```python
from build123d import *

# Parameters (mm, degrees)
HOLE_WIZARD_1_D           = 17.5
HOLE_WIZARD_1_DEPTH       = 23.999
HOLE_WIZARD_1_CSINK_D     = 22.5
HOLE_WIZARD_1_CSINK_ANGLE = 90
SKETCH_4_OUTSIDE_W        = 48.246
SKETCH_4_OUTSIDE_H        = 48.246
CUT_EXTRUDE_1_DEPTH       = 53.473802988


with BuildPart() as part:
    # Эскиз1 → Повернуть1 (revolve)
    with BuildSketch(Plane.XY, mode=Mode.PRIVATE) as revolve_1_sk:
        with BuildLine():
            Line((30.6, 6.5), (33.792893219, 6.5))
            ThreePointArc((33.792893219, 6.5), (33.984234935, 6.538060234), (34.146446609, 6.646446609))
            Line((34.146446609, 6.646446609), (35.5, 8))
            Line((35.5, 8), (45, 8))
            Line((45, 8), (47, 6))
            Line((47, 6), (47, 4))
            Line((47, 4), (26, 4))
            Line((26, 4), (24, 6))
            Line((24, 6), (24, 8.9))
            ThreePointArc((24, 8.9), (23.53137085, 10.03137085), (22.4, 10.5))
            Line((22.4, 10.5), (19.207106781, 10.5))
            ThreePointArc((19.207106781, 10.5), (19.015765065, 10.461939766), (18.853553391, 10.353553391))
            Line((18.853553391, 10.353553391), (8.5, 0))
            Line((8.5, 0), (0, 0))
            Line((0, 0), (0, 12.5))
            Line((0, 12.5), (2.309401077, 16.5))
            Line((2.309401077, 16.5), (26.690598923, 16.5))
            Line((26.690598923, 16.5), (29, 12.5))
            Line((29, 12.5), (29, 8.1))
            ThreePointArc((29, 8.1), (29.46862915, 6.96862915), (30.6, 6.5))
        make_face()
    revolve(revolve_1_sk.sketch.rotate(Axis((-14.464864865, 0, 0), (1, 0, 0)), 90), axis=Axis((-14.464864865, 0, 0), (1, 0, 0)))

    # Отверстие обработанное метчиком 1
    with Locations(Plane.ZY):
        with Locations((0, 0)):
            CounterSinkHole(HOLE_WIZARD_1_D / 2, HOLE_WIZARD_1_CSINK_D / 2, depth=HOLE_WIZARD_1_DEPTH, counter_sink_angle=HOLE_WIZARD_1_CSINK_ANGLE)

    # Эскиз4 outside → Вырез-Вытянуть1 (cut, through all)
    with BuildSketch(Plane.ZY):
        Rectangle(SKETCH_4_OUTSIDE_W, SKETCH_4_OUTSIDE_H)
        Polygon((0, 17.320508076), (-15, 8.660254038), (-15, -8.660254038), (0, -17.320508076), (15, -8.660254038), (15, 8.660254038), align=None, mode=Mode.SUBTRACT)
    extrude(amount=-CUT_EXTRUDE_1_DEPTH, mode=Mode.SUBTRACT)


solid = part.part
```
Input: part model. Units: mm. Frame: model coordinates. A direction names the side the tool comes from. Coordinates: 2 decimals unless noted, no trailing zeros. Loops run counter-clockwise (first coordinate to the right, second up) from the corner with the lowest first, then second, coordinate; pieces in that order, holes last. Notation, with made-up numbers: M -6.75,32 L 26.25,32 A21 cw 26.25,49 Z; hole C 50.25,3.5 d6. An arc over 180 degrees is marked long. Answer in a Markdown table with one row per item.
1. Draft query along Z for faces 1 (the cylindrical face through (14.67, -8.23, 14.3)), 2 (the cylindrical face through (36.353, 3.905, -0.867)), 3 (the cylindrical face through (14.7, -16.5, 0)). Return one class per face: pulls with the +Z half, pulls with the -Z half, needs draft (parallel to the pull), parting line crosses it, or undercut.
Response:
| item | result |
|---|---|
| face 1 | pulls with the +Z half |
| face 2 | undercut |
| face 3 | parting line crosses it |
2. Section A-A, the plane x = 10. Output: boundary loops of the cut face in (y, z).
Response:
| item | result |
|---|---|
| outline | M -16.43,-1.55 L -9.55,-13.45 A16.5 ccw -6.87,-15 L 6.87,-15 A16.5 ccw 9.55,-13.45 L 16.43,-1.55 A16.5 ccw 16.43,1.55 L 9.55,13.45 A16.5 ccw 6.87,15 L -6.87,15 A16.5 ccw -9.55,13.45 L -16.43,1.55 A16.5 ccw Z; hole C 0,0 d17.5 |
3. Reachability of faces 4 (the flat face through (14.317, -12.942, -7.583)), 5 (the cylindrical face through (32.219, 3.955, -5.158)), 6 (the cylindrical face through (9.978, -5.324, 6.944)) from +Z, -Z, +X, -X, +Y, -Y: full face, straight path, thin tool, end or side. Return the list, or none.
Response:
| item | result |
|---|---|
| face 4 | -Z, +X, -X, -Y |
| face 5 | none |
| face 6 | -X |
4. Section B-B, the plane x = 40. Output: boundary loops of the cut face in (y, z), then the cut area to 3 significant figures.
Response:
| item | result |
|---|---|
| outline | C 0,0 d16; hole C 0,0 d8 |
| area | 151 mm2 |
5. Material intervals for line 1 (Y direction, x = 10.75, z = 0); line 2 (Y direction, x = 42, z = 0); line 3 (X direction, y = -11.5, z = -1), sorted ascending.
Response:
| item | result |
|---|---|
| line 1 | y = -16.5 to -8.75, 8.75 to 16.5 |
| line 2 | y = -8 to -4, 4 to 8 |
| line 3 | x = 0 to 29 |
6. First-contact query: pin 1 (5 mm diameter, centred on x = 10.5, z = 1.5, fed in from -Y); pin 2 (1 mm diameter, centred on x = 15.5, z = 4, fed in from -Y); pin 3 (5 mm diameter, centred on y = 11, z = 0, fed in from +X); pin 4 (1.5 mm diameter, centred on x = 6, y = 10, fed in from +Z). Flat tips, straight axial feed; report the tip coordinate or a pass-through.
Response:
| item | result |
|---|---|
| pin 1 | stops at y = -16.5 |
| pin 2 | stops at y = -15.3 |
| pin 3 | stops at x = 29 |
| pin 4 | stops at z = 13.66 |
